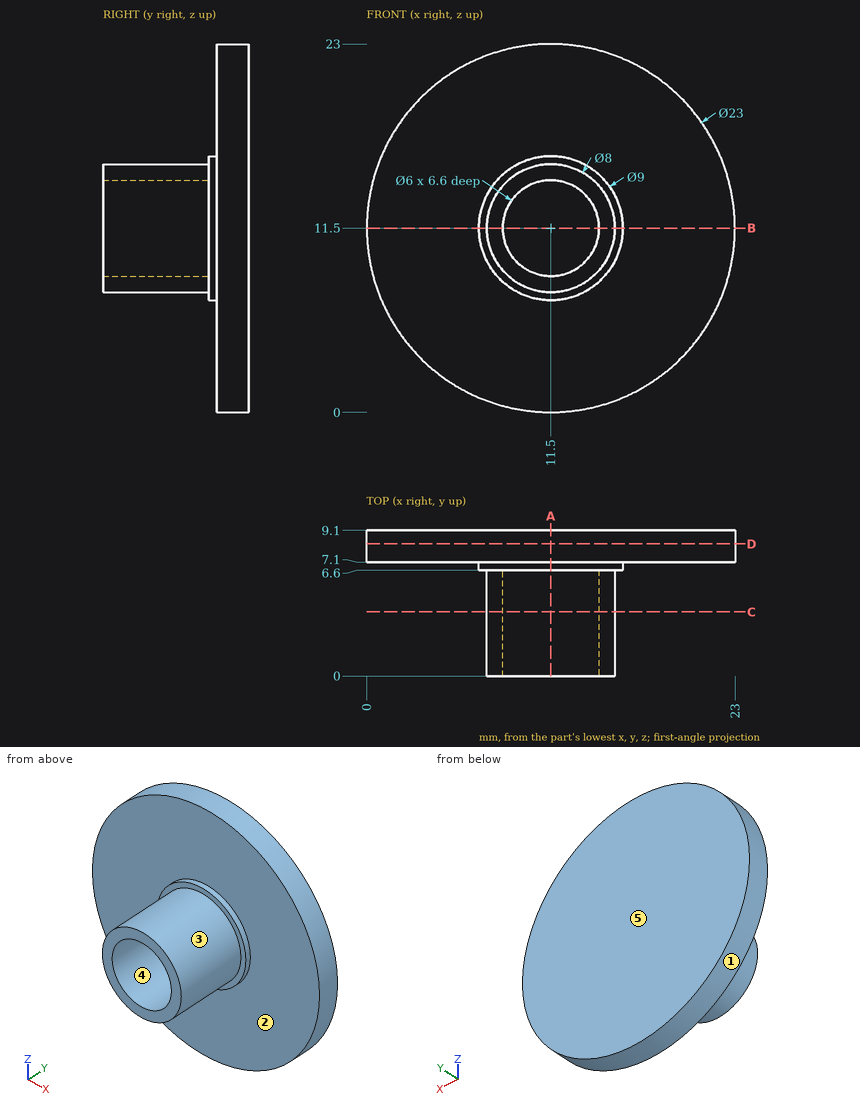
Study the drawing (mm; zero at the part's minimum x, y, z) and answer. A direction names the side the tool comes from. Round coordinates to 2 decimals unless told otherwise and drop trailing zeros. Order: outer loops, then holes, each group sorted by start corner. A loop starts at its lowest first (then second) coordinate and runs counter-clockwise, first axis right, second up. Notation, with made-up numbers: M 47.5,29.25 L 59.5,29.25 A21 cw 59.5,34.25 Z; hole C -21,77 d6. An arc over 180 degrees is marked long. One line per item, written item: value.
Q1. Find section D-D on y = 8.25. Write down the section's boundary in (x, z), then the cut area to 3 significant figures.
Derived:
outline: C 11.5,11.5 d23
area: 415 mm²
Q2. Find section C-C on y = 4. Write down the section's boundary in (x, z), then the cut area to 3 significant figures.
Derived:
outline: C 11.5,11.5 d8; hole C 11.5,11.5 d6
area: 22.0 mm²
Q3. Find section A-A on x = 11.5. Write down the section's boundary in (y, z).
Derived:
outline: M 0,7.5 L 6.6,7.5 L 6.6,7 L 7.1,7 L 7.1,0 L 9.1,0 L 9.1,23 L 7.1,23 L 7.1,16 L 6.6,16 L 6.6,15.5 L 0,15.5 L 0,14.5 L 6.6,14.5 L 6.6,8.5 L 0,8.5 Z
Q4. Straight lines are drawn through the part: line 1 (X direction, y = 3.5, z = 11.5); line 2 (Y direction, x = 21.25, z = 15). For each, find the intervals that lie inside material, in ascending order.
Derived:
line 1: 7.5 to 8.5, 14.5 to 15.5
line 2: 7.1 to 9.1
Q5. Flat-ended cylindrical pins translate along their axes: pin 1 (2.5 mm diameter, centred on x = 12.5, z = 12, fed in from -Y); pin 2 (4 mm diameter, centred on y = 7, z = 9, fed in from +X); pin 3 (3 mm diameter, centred on x = 15, y = 3.5, fed in from +Z). Find the tip coordinate at first contact, or state that the pin passes through.
Derived:
pin 1: y = 6.6
pin 2: x = 22.99
pin 3: z = 14.96
Q6. Find section B-B on z = 11.5. Write down the section's boundary in (x, y).
Derived:
outline: M 0,7.1 L 7,7.1 L 7,6.6 L 7.5,6.6 L 7.5,0 L 8.5,0 L 8.5,6.6 L 14.5,6.6 L 14.5,0 L 15.5,0 L 15.5,6.6 L 16,6.6 L 16,7.1 L 23,7.1 L 23,9.1 L 0,9.1 Z
Q7. For the marked faces 1 and 2, determine the directions among +Z, -Z, +X, -X, +Y, -Y from which every point of the face is accessible in a straight line to the end or side of a thin tool.
Derived:
face 1: +Y, -Y
face 2: -Y
Q8. Determine the mould class of the marked faces 3, 4 and 5 for opening direction X: released by +X, released by -X, zero draft, split by the parting line, or undercut.
Derived:
face 3: split by the parting line
face 4: undercut
face 5: zero draft
